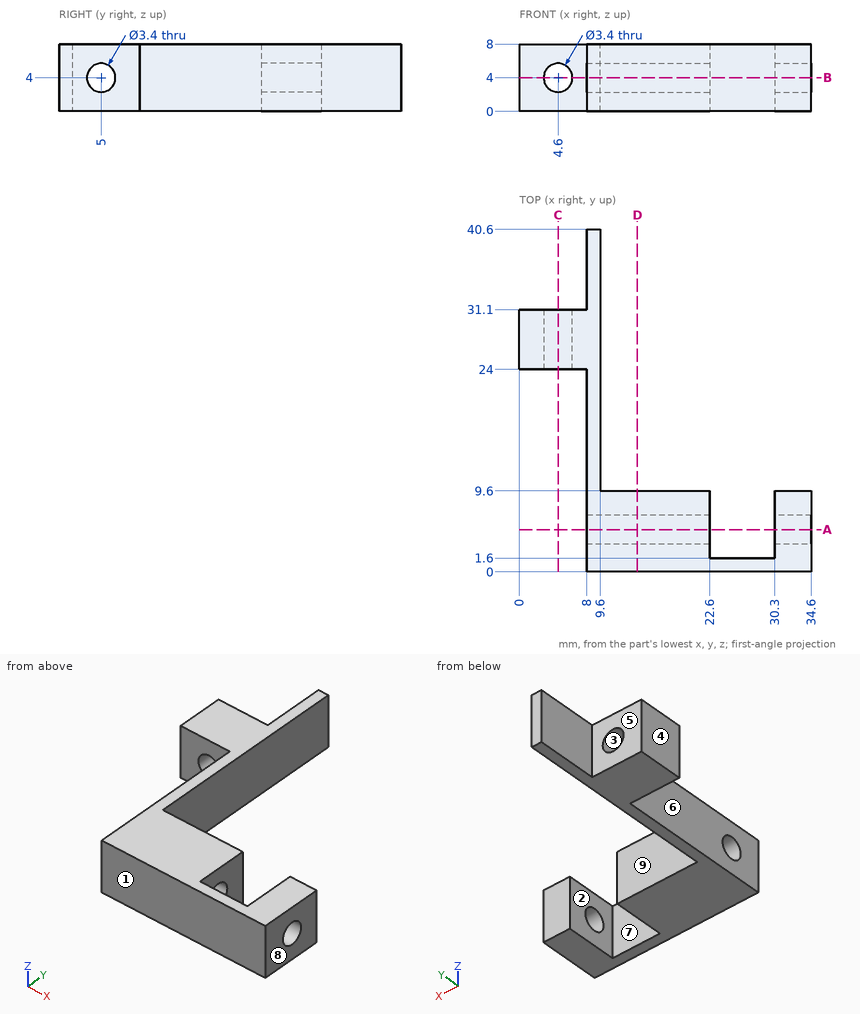
Can you work these out from the drawing? Everything is in mm from the part's minimum corner. A direction names the side the tool comes from. Coordinates: 2 decimals unless noted, no trailing zeros. Loops run counter-clockwise (first coordinate to the right, second up) from the corner with the lowest first, then second, coordinate; pieces in that order, holes last.
1) Imagine slicing it at B-B on z = 4. List the corners of the cut face in (x, y) for me, plus the area to 3 significant figures.
2) Which directions (+Z, -Z, +X, -X, +Y, -Y) give clear straight access to the entire face, cutting with the end or side of a thin tool? Please do the marked faces 5, 6, 7, 8 and 9.
3) Thinking about a two-plate mould opening in X: for the marked faces 1, 2, 3 and 4, which applies, pulls with the +X half, pulls with the -X half, needs draft (parallel to the pull), parting line crosses it, or undercut?
4) I need wall thicknesses on probe 1 along Z at (x, y) = (31.85, 5); probe 2 along X at (y, z) = (3.5, 0.5); probe 3 along X at (y, z) = (34.5, 2.25). Which ranges of each line are inside material? Lowest first, please.
5) Imagine slicing it at A-A on y = 5. List the corners of the cut face in (x, z) for me, plus the area to 3 significant figures.
6) Imagine slicing it at D-D on x = 14. List the corners of the cut face in (y, z) for me, plus the area to 3 significant figures.
7) Imagine slicing it at C-C on x = 4.6. List the corners of the cut face in (y, z) for me, plus the area to 3 significant figures.
8) For pin 1 (2.5 mm diameter, centred on x = 17.5, z = 3.5, fed in from +Y); pin 2 (4 mm diameter, centred on y = 10, z = 2.5, fed in from -X); pin 3 (1 mm diameter, centred on y = 24.5, z = 1.5, fed in from +X); pin 4 (12 mm diameter, centred on x = 20.5, y = 20.5, fed in from -Z), each with a flat end and sliding along its axis, tell me the tip position at first contact or that it passes through.
Completed:
1. outline: (0, 24) - (2.9, 24) - (2.9, 31.1) - (0, 31.1) - close; (6.3, 24) - (8, 24) - (8, 6.7) - (22.6, 6.7) - (22.6, 9.6) - (9.6, 9.6) - (9.6, 40.6) - (8, 40.6) - (8, 31.1) - (6.3, 31.1) - close; (8, 0) - (34.6, 0) - (34.6, 3.3) - (30.3, 3.3) - (30.3, 1.6) - (22.6, 1.6) - (22.6, 3.3) - (8, 3.3) - close; (30.3, 6.7) - (34.6, 6.7) - (34.6, 9.6) - (30.3, 9.6) - close
1. area: 212 mm2
2. face 5: +Z, -Z, -X, +Y
2. face 6: +Z, -Z, -X, -Y
2. face 7: +Z, -Z, +Y
2. face 8: +Z, -Z, +X, +Y, -Y
2. face 9: +Z, -Z, +X, +Y
3. face 1: needs draft
3. face 2: undercut
3. face 3: undercut
3. face 4: pulls with the -X half
4. probe 1: z = 0 to 2.3, 5.7 to 8
4. probe 2: x = 8 to 22.6, 30.3 to 34.6
4. probe 3: x = 8 to 9.6
5. outline: (8, 0) - (22.6, 0) - (22.6, 2.3) - (8, 2.3) - close; (8, 5.7) - (22.6, 5.7) - (22.6, 8) - (8, 8) - close; (30.3, 0) - (34.6, 0) - (34.6, 2.3) - (30.3, 2.3) - close; (30.3, 5.7) - (34.6, 5.7) - (34.6, 8) - (30.3, 8) - close
5. area: 86.9 mm2
6. outline: (0, 0) - (9.6, 0) - (9.6, 8) - (0, 8) - close; hole circle Ø3.4 at (5, 4)
6. area: 67.7 mm2
7. outline: (24, 0) - (31.1, 0) - (31.1, 2.3) - (24, 2.3) - close; (24, 5.7) - (31.1, 5.7) - (31.1, 8) - (24, 8) - close
7. area: 32.7 mm2
8. pin 1: stops at y = 9.6
8. pin 2: stops at x = 8
8. pin 3: stops at x = 9.6
8. pin 4: passes through
